```python
from build123d import *

# Parameters (mm, degrees)
SZKIC1_R                    = 1.15
DODANIE_WYCI_GNI_CIE1_DEPTH = 2


with BuildPart() as part:
    # Szkic1 → Dodanie-wyciągnięcie1 (new body)
    with BuildSketch(Plane.XY):
        with BuildLine():
            Line((-5.8, -4.994143627), (5.8, -4.994143627))
            Line((5.8, -4.994143627), (5.8, 0.63488027))
            ThreePointArc((5.8, 0.63488027), (5.10760912, 2.994496299), (3.25, 4.605856373))
            Line((3.25, 4.605856373), (-3.25, 4.605856373))
            ThreePointArc((-3.25, 4.605856373), (-5.10760912, 2.994496299), (-5.8, 0.63488027))
            Line((-5.8, 0.63488027), (-5.8, -4.994143627))
        make_face()
        Circle(SZKIC1_R, mode=Mode.SUBTRACT)
        with Locations((3.5, 0)):
            Circle(SZKIC1_R, mode=Mode.SUBTRACT)
        with Locations((-3.5, 0)):
            Circle(SZKIC1_R, mode=Mode.SUBTRACT)
    extrude(amount=DODANIE_WYCI_GNI_CIE1_DEPTH)


solid = part.part
```
Read the model definition and answer for the solid it produces. Units are mm, in the model's axes. Give positions to 0.01 mm unless a question says otherwise; leave off trailing zeros. Order: outer loops, then holes, each group sorted by start corner. A loop starts at its lowest first (then second) coordinate and runs counter-clockwise, first axis right, second up. Notation, with made-up numbers: (42, 39) -> (72, 39) arc R13 cw to (72, 48) -> close; hole circle Ø10 at (72.25, 71). An arc over 180 degrees is marked (long way). One line per item, written item: value. Start each with the question number.
(1) Flat-ended cylindrical pins translate along their axes: P1, Ø2.5, axis at x = 0, y = 0, coming from the -Z side; P2, Ø1.8, axis at x = -3.5, y = 0, coming from the -Z side; P3, Ø1, axis at x = -4.5, z = 1, coming from the +Y side. Find the tip coordinate at first contact, or state that the pin passes through.
(2) Straight lines are drawn through the part: L1, parallel to Y at x = 0, z = 1.6; L2, parallel to X at y = -0.5, z = 0.45; L3, parallel to X at y = -1, z = 0.7. For each, find the intervals that lie inside material, in ascending order.
(3) The part is cut by section A-A (x = 0). Determine the outline of the cut face in (y, z), and give its area (3 significant figures).
(4) The part is cut by section B-B (z = 1.7). Determine the outline of the cut face in (x, y).
(5) The part is cut by section C-C (y = 0). Determine the outline of the cut face in (x, z).
(6) For a pull along X with two mould halves and no side action, classify faces 1 (the cylindrical face through (-3.749, -1.123, 0.986)), 2 (the cylindrical face through (3.251, -1.123, 0.986)), 3 (the cylindrical face through (5.126, 2.965, 0.986)), 4 (the flat face through (-5.8, -2, 1)) as released by +X, released by -X, zero draft, split by the parting line, or undercut.
(7) The part is cut by section D-D (x = -3.5). Determine the outline of the cut face in (y, z), and give its area (3 significant figures).
Taken from the geometry:
1. P1: z = 0
1. P2: through
1. P3: y = 4.17
2. L1: -4.99 to -1.15, 1.15 to 4.61
2. L2: -5.8 to -4.54, -2.46 to -1.04, 1.04 to 2.46, 4.54 to 5.8
2. L3: -5.8 to -4.07, -2.93 to -0.57, 0.57 to 2.93, 4.07 to 5.8
3. outline: (-4.99, 0) -> (-1.15, 0) -> (-1.15, 2) -> (-4.99, 2) -> close; (1.15, 0) -> (4.61, 0) -> (4.61, 2) -> (1.15, 2) -> close
3. area: 14.6 mm^2
4. outline: (-5.8, -4.99) -> (5.8, -4.99) -> (5.8, 0.63) arc R4.37 ccw to (3.25, 4.61) -> (-3.25, 4.61) arc R4.37 ccw to (-5.8, 0.63) -> close; hole circle Ø2.3 at (-3.5, 0); hole circle Ø2.3 at (0, 0); hole circle Ø2.3 at (3.5, 0)
5. outline: (-5.8, 0) -> (-4.65, 0) -> (-4.65, 2) -> (-5.8, 2) -> close; (-2.35, 0) -> (-1.15, 0) -> (-1.15, 2) -> (-2.35, 2) -> close; (1.15, 0) -> (2.35, 0) -> (2.35, 2) -> (1.15, 2) -> close; (4.65, 0) -> (5.8, 0) -> (5.8, 2) -> (4.65, 2) -> close
6. face 1: undercut
6. face 2: undercut
6. face 3: released by +X
6. face 4: released by -X
7. outline: (-4.99, 0) -> (-1.15, 0) -> (-1.15, 2) -> (-4.99, 2) -> close; (1.15, 0) -> (4.48, 0) -> (4.48, 2) -> (1.15, 2) -> close
7. area: 14.4 mm^2
